from build123d import *

# Parameters (mm, degrees)
SKETCH1_W           = 57.15
SKETCH1_H           = 19.05
BOSS_EXTRUDE1_DEPTH = 3.175
SKETCH2_W           = 57.15
SKETCH2_H           = 6.398717948
BOSS_EXTRUDE2_DEPTH = 19.05
FILLET1_R           = 2.54


with BuildPart() as part:
    # Sketch1 → Boss-Extrude1 (new body)
    with BuildSketch(Plane.XY):
        Rectangle(SKETCH1_W, SKETCH1_H)
    extrude(amount=BOSS_EXTRUDE1_DEPTH)

    # Sketch2 → Boss-Extrude2 (add)
    with BuildSketch(Plane.XY.offset(3.175)):
        Rectangle(SKETCH2_W, SKETCH2_H)
    extrude(amount=BOSS_EXTRUDE2_DEPTH)

    # Fillet1
    fillet1_edges = [part.edges().sort_by_distance(p)[0] for p in [
        (28.575, -9.525, 1.5875),
        (-28.575, -9.525, 1.5875),
        (-28.575, 9.525, 1.5875),
        (28.575, 9.525, 1.5875),
    ]]
    fillet(fillet1_edges, radius=FILLET1_R)


solid = part.part
Model file for the job. Use its own axes, mm. A direction names the side the tool comes from. Round coordinates to 2 decimals unless told otherwise and drop trailing zeros. Order: outer loops, then holes, each group sorted by start corner. A loop starts at its lowest first (then second) coordinate and runs counter-clockwise, first axis right, second up.
(1) Band-saw the part on C-C (y = 3.75). List the corners of the cut face in (x, z) (3 decimals).
(2) Drill centre lines: line 1 (Y direction, x = 25.5, z = 11.25); line 2 (Z direction, x = 1.5, y = -5.5) (3 decimals). Where is each one in solid material? Low to high.
(3) Pin check, flat tips, straight feed: pin 1 (5.5 mm diameter, centred on x = -7, z = 9.5, fed in from +Y); pin 2 (7 mm diameter, centred on x = 1, y = 6, fed in from +Z) (3 decimals); pin 3 (4 mm diameter, centred on x = -7.5, z = 5.5, fed in from -Y); pin 4 (3 mm diameter, centred on x = -12.5, y = -8, fed in from +Z) (3 decimals). Stop position of each tip, or through.
(4) 3-axis set-ups, long thin cutter, end or side, ignore diameter. For faces 1 (the face through (0, 3.199, 13)), 2 (the face through (0, 0, 0)), 3 (the face through (0, -6, 3.175)): which of +Z, -Z, +X, -X, +Y, -Y reach the whole face in a straight line?
(5) Band-saw the part on A-A (x = -13). List the corners of the cut face in (y, z) (3 decimals), then the cut area to 3 significant figures.
(6) Band-saw the part on B-B (z = 16.5). List the corners of the cut face in (x, y) (3 decimals).
Verdict:
1. outline: (-28.575, 0) - (28.575, 0) - (28.575, 3.175) - (-28.575, 3.175) - close
2. line 1: y = -3.2 to 3.2
2. line 2: z = 0 to 3.175
3. pin 1: stops at y = 3.2
3. pin 2: stops at z = 22.225
3. pin 3: stops at y = -3.2
3. pin 4: stops at z = 3.175
4. face 1: +Z, +X, -X, +Y
4. face 2: -Z, +X, -X, +Y, -Y
4. face 3: +Z, +X, -X, -Y
5. outline: (-9.525, 0) - (9.525, 0) - (9.525, 3.175) - (3.199, 3.175) - (3.199, 22.225) - (-3.199, 22.225) - (-3.199, 3.175) - (-9.525, 3.175) - close
5. area: 182 mm2
6. outline: (-28.575, -3.199) - (28.575, -3.199) - (28.575, 3.199) - (-28.575, 3.199) - close
